Source: CAD feature listing. Evaluate the final solid. Frame: model axes, mm. A direction names the side the tool comes from. Coordinates: 2 decimals unless noted, no trailing zeros. Write each loop counter-clockwise with the first axis right and the second up, starting at its lowest first coordinate (ties: lowest second). Pieces come first, ordered by that corner, then holes. Notation, with made-up numbers: (-24, 43) - (-11, 43) arc R20 cw to (-11, 47) - close; hole circle Ø8 at (-6, 8). An arc over 180 degrees is marked (long way). One line per item, written item: value.
from build123d import *

# Parameters (mm, degrees)
SKETCH1_W           = 28
SKETCH1_H           = 16
BOSS_EXTRUDE1_DEPTH = 10
CUT_EXTRUDE1_REACH  = 12
SKETCH2_R           = 1.5
SKETCH3_W           = 22.631801359
SKETCH3_H           = 10
BOSS_EXTRUDE2_DEPTH = 2


with BuildPart() as part:
    # Sketch1 → Boss-Extrude1 (new body)
    with BuildSketch(Plane(origin=(0, 0, 0), x_dir=(1, 0, 0), z_dir=(0, 1, 0))):
        Rectangle(SKETCH1_W, SKETCH1_H)
    extrude(amount=BOSS_EXTRUDE1_DEPTH)

    # Sketch2 → Cut-Extrude1 (cut, up to next)
    with BuildSketch(Plane(origin=(0, 10, 0), x_dir=(1, 0, 0), z_dir=(0, 1, 0)), mode=Mode.PRIVATE) as cut_extrude1_sk1:
        with Locations((-11.3, -5.3)):
            Circle(SKETCH2_R)
    cut_extrude1_tool1 = extrude(cut_extrude1_sk1.sketch, amount=-CUT_EXTRUDE1_REACH, mode=Mode.PRIVATE) & part.part
    add(cut_extrude1_tool1.solids().sort_by_distance((-11.3, 10, 5.3))[0], mode=Mode.SUBTRACT)
    # Sketch2 → Cut-Extrude1 (cut, up to next)
    with BuildSketch(Plane(origin=(0, 10, 0), x_dir=(1, 0, 0), z_dir=(0, 1, 0)), mode=Mode.PRIVATE) as cut_extrude1_sk2:
        with Locations((11.3, 5.3)):
            Circle(SKETCH2_R)
    cut_extrude1_tool2 = extrude(cut_extrude1_sk2.sketch, amount=-CUT_EXTRUDE1_REACH, mode=Mode.PRIVATE) & part.part
    add(cut_extrude1_tool2.solids().sort_by_distance((11.3, 10, -5.3))[0], mode=Mode.SUBTRACT)

    # Sketch3 → Boss-Extrude2 (add)
    with BuildSketch(Plane.XY.offset(8)):
        with Locations((12.68409932, 5)):
            Rectangle(SKETCH3_W, SKETCH3_H)
    extrude(amount=BOSS_EXTRUDE2_DEPTH)


solid = part.part
1) Section query D-D on z = 0. Output: boundary loops of the cut face in (x, y), then the cut area to 3 significant figures.
Values found:
outline: (-14, 0) - (14, 0) - (14, 10) - (-14, 10) - close
area: 280 mm2
2) Reachability of faces 5 (the flat face through (14, 5, 0)), 6 (the cylindrical face through (12.73, 5.07, -5.75)), 7 (the flat face through (1.368, 5, 9)) from +Z, -Z, +X, -X, +Y, -Y: full face, straight path, thin tool, end or side. Return the list, or none.
Values found:
face 5: -Z, +X, +Y, -Y
face 6: +Y, -Y
face 7: +Z, -X, +Y, -Y
3) Section query C-C on y = 7.5. Output: boundary loops of the cut face in (x, z), then the cut area to 3 significant figures.
Values found:
outline: (-14, -8) - (14, -8) - (14, 8) - (24, 8) - (24, 10) - (1.37, 10) - (1.37, 8) - (-14, 8) - close; hole circle Ø3 at (-11.3, 5.3); hole circle Ø3 at (11.3, -5.3)
area: 479 mm2
4) Contact query for flat-ended pins moving along their axis: P1, Ø0.6, axis at y = 3.5, z = 9.5, coming from the -X side; P2, Ø2.5, axis at x = 11.3, z = -5.3, coming from the +Y side; P3, Ø3, axis at x = -3.5, y = 5, coming from the +Z side; P4, Ø4, axis at y = 2.5, z = -3, coming from the +X side. Output: stop coordinate, or through.
Values found:
P1: x = 1.37
P2: through
P3: z = 8
P4: x = 14
5) Section query B-B on z = 5.3. Output: boundary loops of the cut face in (x, y).
Values found:
outline: (-14, 0) - (-12.8, 0) - (-12.8, 10) - (-14, 10) - close; (-9.8, 0) - (14, 0) - (14, 10) - (-9.8, 10) - close
6) Material intervals for line 1 (X direction, y = 4.25, z = 5.3); line 2 (Z direction, x = -11.3, y = 2.5); line 3 (Z direction, x = 11.3, y = 3.5), sorted ascending.
Values found:
line 1: -14 to -12.8, -9.8 to 14
line 2: -8 to 3.8, 6.8 to 8
line 3: -8 to -6.8, -3.8 to 10
7) Section query A-A on x = 11.3. Output: boundary loops of the cut face in (y, z).
Values found:
outline: (0, -8) - (10, -8) - (10, -6.8) - (0, -6.8) - close; (0, -3.8) - (10, -3.8) - (10, 10) - (0, 10) - close
8) Draft query along Z for faces 1 (the flat face through (13, 5, 10)), 2 (the flat face through (19, 5, 8)), 3 (the flat face through (-14, 5, 0)), 4 (the cylindrical face through (-12.8, 5.07, 5.23)). Return one class per face: released by +Z, released by -Z, zero draft, split by the parting line, or undercut.
Values found:
face 1: released by +Z
face 2: released by -Z
face 3: zero draft
face 4: undercut
